Model file for the job. Use its own axes, mm. A direction names the side the tool comes from. Round coordinates to 2 decimals unless told otherwise and drop trailing zeros. Order: outer loops, then holes, each group sorted by start corner. A loop starts at its lowest first (then second) coordinate and runs counter-clockwise, first axis right, second up. Notation, with made-up numbers: (-0.75, -10) -> (28.25, -10) arc R21 ccw to (28.25, 24) -> close; hole circle Ø11 at (39, 55.5). An arc over 180 degrees is marked (long way). Answer as CSV lines item,"result".
```python
from build123d import *

# Parameters (mm, degrees)
F1_DEPTH = 6


with BuildPart() as f1:
    # F0 (on Top) → F1 (new body)
    with BuildSketch(Plane.XY):
        with BuildLine():
            ThreePointArc((-39.53987, 13.785708), (-37.782511, 9.543067), (-33.53987, 7.785708))
            Line((-33.53987, 7.785708), (14.46013, 7.785708))
            ThreePointArc((14.46013, 7.785708), (18.702771, 9.543067), (20.46013, 13.785708))
            Line((20.46013, 13.785708), (20.46013, 19.785708))
            ThreePointArc((20.46013, 19.785708), (18.702771, 24.028348), (14.46013, 25.785708))
            Line((14.46013, 25.785708), (-33.53987, 25.785708))
            ThreePointArc((-33.53987, 25.785708), (-37.782511, 24.028348), (-39.53987, 19.785708))
            Line((-39.53987, 19.785708), (-39.53987, 13.785708))
        make_face()
        with BuildLine():
            Line((11.46013, 13.785708), (-30.53987, 13.785708))
            ThreePointArc((-30.53987, 13.785708), (-33.53987, 16.785708), (-30.53987, 19.785708))
            Line((-30.53987, 19.785708), (11.46013, 19.785708))
            ThreePointArc((11.46013, 19.785708), (14.46013, 16.785708), (11.46013, 13.785708))
        make_face(mode=Mode.SUBTRACT)
    extrude(amount=F1_DEPTH)


solid = f1.part
```
Q1. Saw through at B-B (x = -8.5). Write the cut outline in (y, z).
Checks:
outline,"(7.79, 0) -> (13.79, 0) -> (13.79, 6) -> (7.79, 6) -> close; (19.79, 0) -> (25.79, 0) -> (25.79, 6) -> (19.79, 6) -> close"
Q2. Wall check: L1, parallel to Y at x = 6.5, z = 2.75; L2, parallel to X at y = 17.25, z = 5.5; L3, parallel to X at y = 14.5, z = 3. Give the ranges that are in metal, low to high. Write a range as [from, to].
Checks:
L1,"[7.79, 13.79], [19.79, 25.79]"
L2,"[-39.54, -33.5], [14.42, 20.46]"
L3,"[-39.54, -32.48], [13.4, 20.46]"
Q3. Saw through at A-A (z = 2.4). Write the cut outline in (x, y).
Checks:
outline,"(-39.54, 13.79) arc R6 ccw to (-33.54, 7.79) -> (14.46, 7.79) arc R6 ccw to (20.46, 13.79) -> (20.46, 19.79) arc R6 ccw to (14.46, 25.79) -> (-33.54, 25.79) arc R6 ccw to (-39.54, 19.79) -> close; hole (-30.54, 13.79) -> (11.46, 13.79) arc R3 ccw to (11.46, 19.79) -> (-30.54, 19.79) arc R3 ccw to start"
Q4. Flat gauge pin, fed straight in: pin 1 (3 mm diameter, centred on y = 11, z = 4.5, fed in from -X). Where does the tip first touch, or does it go through?
Checks:
pin 1,"x = -39.4"
Q5. Saw through at C-C (y = 18.75). Write the cut outline in (x, z).
Checks:
outline,"(-39.54, 0) -> (-32.81, 0) -> (-32.81, 6) -> (-39.54, 6) -> close; (13.73, 0) -> (20.46, 0) -> (20.46, 6) -> (13.73, 6) -> close"
Q6. Tool access for faces 1 (the flat face through (-10, 19.786, 3)), 2 (the cylindrical face through (-37.74, 24.07, 2.96)): list every direction of +Z, -Z, +X, -X, +Y, -Y with a clear straight run to the whole face (end or side of a thin tool).
Checks:
face 1,"+Z, -Z"
face 2,"+Z, -Z, -X, +Y"
Q7. Mould opens along X. For faces 3 (the flat face through (-39.54, 17, 3)), 4 (the flat face through (-9, 25.786, 3)), 5 (the flat face through (-9, 13.786, 3)) say: +X half, -X half, draft (parallel to the pull), parting line (faces both ways), or undercut.
Checks:
face 3,"-X half"
face 4,"draft"
face 5,"undercut"
Q8. Saw through at D-D (y = 9.5). Write the cut outline in (x, z).
Checks:
outline,"(-37.74, 0) -> (18.66, 0) -> (18.66, 6) -> (-37.74, 6) -> close"
